Here's how the part is built. I have some questions about the finished solid (model axes, mm). Face numbers are marked on the shaded views. A direction names the side the tool comes from. Round coordinates to 2 decimals unless told otherwise and drop trailing zeros. Write each loop counter-clockwise with the first axis right and the second up, starting at its lowest first coordinate (ties: lowest second). Pieces come first, ordered by that corner, then holes. Notation, with made-up numbers: (75, 49) -> (106, 49) arc R17 cw to (106, 67) -> close; hole circle Ø3 at (59, 28.5). An arc over 180 degrees is marked (long way). Answer in a Markdown table with one row per item.
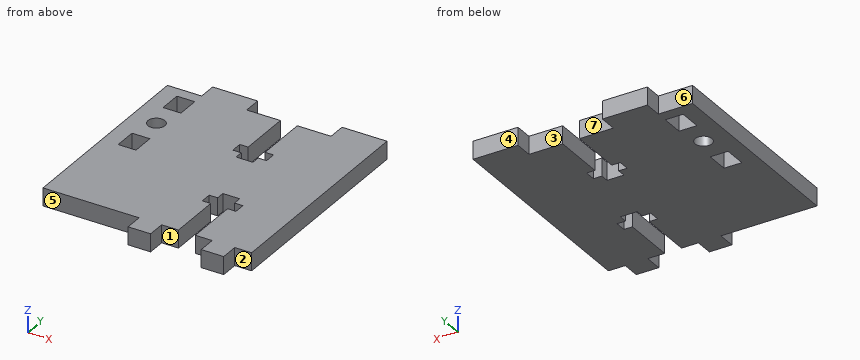
from build123d import *

# Parameters (mm, degrees)
F0_W     = 3.175
F0_H     = 4
F0_R     = 1.5
F1_DEPTH = 3.175


# Not quite as in the source:
# - a length typed as a fraction of an inch, garbled in the dataset ("3 / 203.2 mm" for 3/8 in), is restored
# - a feature names something its author has since deleted; it is built from what else it names


with BuildPart() as f1:
    # F0 (on Top) → F1 (new body)
    with BuildSketch(Plane.XY):
        Polygon((11.1548891366, 23.9696219414), (8.1548891366, 23.9696219414), (8.1548891366, 25.4696219414), (6.6548891366, 25.4696219414), (6.6548891366, 27.4696219414), (8.1548891366, 27.4696219414), (8.1548891366, 36.7946219414), (2.1548891366, 36.7946219414), (2.1548891366, 39.9696219414), (-5.8451108634, 39.9696219414), (-5.8451108634, 36.7946219414), (-11.9326108634, 36.7946219414), (-11.9326108634, 0.7946219414), (5.1548891366, 0.7946219414), (5.1548891366, -2.3803780586), (9.1548891366, -2.3803780586), (9.1548891366, 0.7946219414), (12.1548891366, 0.7946219414), (12.1548891366, 10.1196219414), (10.6548891366, 10.1196219414), (10.6548891366, 12.1196219414), (12.1548891366, 12.1196219414), (12.1548891366, 13.6196219414), (15.1548891366, 13.6196219414), (15.1548891366, 12.1196219414), (16.6548891366, 12.1196219414), (16.6548891366, 10.1196219414), (15.1548891366, 10.1196219414), (15.1548891366, 0.7946219414), (18.1548891366, 0.7946219414), (18.1548891366, -2.3803780586), (22.1548891366, -2.3803780586), (22.1548891366, 0.7946219414), (25.1548891366, 0.7946219414), (25.1548891366, 36.7946219414), (25.1548891366, 39.9696219414), (17.1548891366, 39.9696219414), (17.1548891366, 36.7946219414), (11.1548891366, 36.7946219414), (11.1548891366, 27.4696219414), (12.6548891366, 27.4696219414), (12.6548891366, 25.4696219414), (11.1548891366, 25.4696219414), align=None)
        with Locations((-7.4326108634, 19.7946219414)):
            Rectangle(F0_W, F0_H, mode=Mode.SUBTRACT)
        with Locations((-7.4326108634, 26.2946219414)):
            Circle(F0_R, mode=Mode.SUBTRACT)
        with Locations((-7.4326108634, 32.7946219414)):
            Rectangle(F0_W, F0_H, mode=Mode.SUBTRACT)
    extrude(amount=F1_DEPTH)


solid = f1.part
1) I want a section at B-B, the plane y = 11. List the corners of the cut face in (x, z) for me (3 decimals).
Response:
| item | result |
|---|---|
| outline | (-11.933, 0) -> (10.655, 0) -> (10.655, 3.175) -> (-11.933, 3.175) -> close; (16.655, 0) -> (25.155, 0) -> (25.155, 3.175) -> (16.655, 3.175) -> close |
2) I need wall thicknesses on line 1 (X direction, y = 34.5, z = 0.15); line 2 (X direction, y = 37, z = 0.75); line 3 (X direction, y = 12, z = 0.2). Which ranges of each line are inside material? Lowest first, please. Write a range as [from, to].
Response:
| item | result |
|---|---|
| line 1 | x = [-11.93, -9.02], [-5.85, 8.15], [11.15, 25.15] |
| line 2 | x = [-5.85, 2.15], [17.15, 25.15] |
| line 3 | x = [-11.93, 10.65], [16.65, 25.15] |
3) I want a section at D-D, the plane x = 0.5. List the corners of the cut face in (y, z) for me (3 decimals).
Response:
| item | result |
|---|---|
| outline | (0.795, 0) -> (39.97, 0) -> (39.97, 3.175) -> (0.795, 3.175) -> close |
4) For pin 1 (1.5 mm diameter, centred on x = 5.5, z = 2.5, fed in from +Y); pin 2 (1.5 mm diameter, centred on x = 9, z = 1.5, fed in from +Y); pin 3 (1 mm diameter, centred on y = -1.5, z = 1.5, fed in from +X), each with a flat end and sliding along its axis, tell me the tip position at first contact or that it passes through.
Response:
| item | result |
|---|---|
| pin 1 | stops at y = 36.79 |
| pin 2 | stops at y = 23.97 |
| pin 3 | stops at x = 22.15 |
5) I want a section at C-C, the plane x = -8. List the corners of the cut face in (y, z) for me (3 decimals).
Response:
| item | result |
|---|---|
| outline | (0.795, 0) -> (17.795, 0) -> (17.795, 3.175) -> (0.795, 3.175) -> close; (21.795, 0) -> (24.906, 0) -> (24.906, 3.175) -> (21.795, 3.175) -> close; (27.683, 0) -> (30.795, 0) -> (30.795, 3.175) -> (27.683, 3.175) -> close; (34.795, 0) -> (36.795, 0) -> (36.795, 3.175) -> (34.795, 3.175) -> close |
6) I want a section at A-A, the plane y = 2.5. List the corners of the cut face in (x, z) for me (3 decimals), and give its area (3 significant figures).
Response:
| item | result |
|---|---|
| outline | (-11.933, 0) -> (12.155, 0) -> (12.155, 3.175) -> (-11.933, 3.175) -> close; (15.155, 0) -> (25.155, 0) -> (25.155, 3.175) -> (15.155, 3.175) -> close |
| area | 108 mm^2 |
7) We'd pull the mould along X, two halves only. Please class the marked faces 1, 2 and 3: +X half, -X half, draft (parallel to the pull), parting line (faces both ways), or undercut.
Response:
| item | result |
|---|---|
| face 1 | undercut |
| face 2 | draft |
| face 3 | undercut |
8) Which directions (+Z, -Z, +X, -X, +Y, -Y) give clear straight access to the entire face, cutting with the end or side of a thin tool? Please do the marked faces 4, 5, 6 and 7.
Response:
| item | result |
|---|---|
| face 4 | +Z, -Z, +X, -X, +Y |
| face 5 | +Z, -Z, -X, -Y |
| face 6 | +Z, -Z, -X, +Y |
| face 7 | +Z, -Z, +Y |
